```python
from build123d import *

# Parameters (mm, degrees)
SKETCH_W          = 102.2
SKETCH_H          = 83
SKETCH_W_2        = 30
SKETCH_H_2        = 5
SKETCH_W_3        = 2
SKETCH_H_3        = 25
PAD_DEPTH         = 2
SKETCH001_R       = 2.4
SKETCH001_R_2     = 1.2
PAD001_DEPTH      = 6.2
PAD002_DEPTH      = 6.9
PAD002_DEPTH_BACK = 2
PAD003_DEPTH      = 1
SKETCH004_W       = 1.45
SKETCH004_H       = 11.2
PAD004_DEPTH      = 7
SKETCH005_W       = 1.45
SKETCH005_H       = 5
PAD005_DEPTH      = 3
PAD006_DEPTH      = 5
SKETCH008_W       = 35.5
SKETCH008_H       = 1
POCKET_DEPTH      = 107.001
SKETCH009_W       = 14
SKETCH009_H       = 1
POCKET001_DEPTH   = 4.5


with BuildPart() as part:
    # Sketch → Pad (new body)
    with BuildSketch(Plane.XY):
        Rectangle(SKETCH_W, SKETCH_H)
        with Locations((34.1, 18.5)):
            Rectangle(SKETCH_W_2, SKETCH_H_2, mode=Mode.SUBTRACT)
        with Locations((6, -27)):
            Rectangle(SKETCH_W_3, SKETCH_H_3, mode=Mode.SUBTRACT)
        with Locations((-34.1, 18.5)):
            Rectangle(SKETCH_W_2, SKETCH_H_2, mode=Mode.SUBTRACT)
        with Locations((-6, -27)):
            Rectangle(SKETCH_W_3, SKETCH_H_3, mode=Mode.SUBTRACT)
    extrude(amount=PAD_DEPTH)

    # Sketch001 (on Face22 of Pad) → Pad001 (join)
    with BuildSketch(Plane.XY.offset(2)):
        with Locations((-42.5, -25)):
            Circle(SKETCH001_R)
        with Locations((-42.5, -25)):
            Circle(SKETCH001_R_2, mode=Mode.SUBTRACT)
        with Locations((42.5, 25)):
            Circle(SKETCH001_R)
        with Locations((42.5, 25)):
            Circle(SKETCH001_R_2, mode=Mode.SUBTRACT)
    extrude(amount=PAD001_DEPTH)

    # Sketch002 (on Face5 of Pad001) → Pad002 (join, two sides)
    with BuildSketch(Plane.XY.offset(2)) as pad002_sk:
        Polygon((51.1, 5), (53.5, 5), (53.5, 43.85), (-53.5, 43.85), (-53.5, 5), (-51.1, 5), (-51.1, 41.5), (51.1, 41.5), align=None)
        Polygon((51.1, -5), (53.5, -5), (53.5, -43.85), (-53.5, -43.85), (-53.5, -5), (-51.1, -5), (-51.1, -41.5), (51.1, -41.5), align=None)
    extrude(amount=PAD002_DEPTH)
    extrude(pad002_sk.sketch, amount=-PAD002_DEPTH_BACK)

    # Sketch003 (on Face33 of Pad002) → Pad003 (join)
    with BuildSketch(Plane.XY.offset(8.9)):
        Polygon((-52.1, 5), (-51.1, 5), (-51.1, 41.5), (51.1, 41.5), (51.1, 5), (52.1, 5), (52.1, 42.5), (-52.1, 42.5), align=None)
        Polygon((-52.1, -5), (-51.1, -5), (-51.1, -41.5), (51.1, -41.5), (51.1, -5), (52.1, -5), (52.1, -42.5), (-52.1, -42.5), align=None)
    extrude(amount=PAD003_DEPTH)

    # Sketch004 (on Face3 of Pad003) → Pad004 (join)
    with BuildSketch(Plane.XY.offset(2)):
        with Locations((50.375, 0)):
            Rectangle(SKETCH004_W, SKETCH004_H)
        with Locations((-50.375, 0)):
            Rectangle(SKETCH004_W, SKETCH004_H)
    extrude(amount=PAD004_DEPTH)

    # Sketch005 (on Face49 of Pad004) → Pad005 (join)
    with BuildSketch(Plane.XY.offset(9)):
        with Locations((50.375, 0)):
            Rectangle(SKETCH005_W, SKETCH005_H)
        with Locations((-50.375, 0)):
            Rectangle(SKETCH005_W, SKETCH005_H)
    extrude(amount=PAD005_DEPTH)

    # Sketch006 (on Face45 of Pad005) → Pad006 (join)
    with BuildSketch(Plane.XZ.offset(2.5)):
        Polygon((-51.10001, 12), (-53.10001, 12), (-53.10001, 13), (-51.15, 16), (-49.65, 16), (-49.65, 12), align=None)
    pad006 = extrude(amount=-PAD006_DEPTH)

    # Mirrored: Pad006 across YZ
    add(pad006.mirror(Plane.YZ))

    # Sketch008 (on Face47 of Mirrored) → Pocket (cut, through all)
    with BuildSketch(Plane.YZ.offset(53.5)):
        with Locations((0, 0.5)):
            Rectangle(SKETCH008_W, SKETCH008_H)
    extrude(amount=-POCKET_DEPTH, mode=Mode.SUBTRACT)

    # Sketch009 (on Face74 of Pocket) → Pocket001 (cut)
    with BuildSketch(Plane.XZ.offset(43.85)):
        with Locations((0, 0.5)):
            Rectangle(SKETCH009_W, SKETCH009_H)
    extrude(amount=-POCKET001_DEPTH, mode=Mode.SUBTRACT)


solid = part.part
```
Read the model definition and answer for the solid it produces. Units are mm, in the model's axes. A direction names the side the tool comes from. Coordinates: 2 decimals unless noted, no trailing zeros. Write each loop counter-clockwise with the first axis right and the second up, starting at its lowest first coordinate (ties: lowest second). Pieces come first, ordered by that corner, then holes. Notation, with made-up numbers: (-19, 5.25) - (38, 5.25) arc R11 cw to (38, 22.25) - close; hole circle Ø1 at (41.5, 35.25). An arc over 180 degrees is marked (long way). Answer as a JSON object with one key per item and string values. Group by question number.
1. A cutting plane is placed at D-D (x = -17.5). Determine the outline of the cut face in (y, z).
2. A cutting plane is placed at B-B (y = -20). Determine the outline of the cut face in (x, z).
3. Which of the six approach directions +Z, -Z, +X, -X, +Y, -Y give full straight-line access (tool end or side, diameter ignored) to faces 1 (the flat face through (1, 0, 1)), 2 (the flat face through (52, -5, 6)), 3 (the flat face through (0, -42, 1)), 4 (the flat face through (51.1, 0, 6)), 5 (the flat face through (41, 25, 8.2))?
4. Consider L1, parallel to Y at x = 42.5, z = 6.25; L2, parallel to Y at x = 19, z = 4.5; L3, parallel to Y at x = 34, z = 9.5. Determine where each line is inside the solid, lowest interval first. Write a range as [from, to].
5. The mould has two halves that part along Y. Classify faces 6 (the flat face through (51.1, -24, 6)), 7 (the flat face through (-31, -31, 0)), 8 (the flat face through (1, -43.85, 5)): +Y half, -Y half, draft (parallel to the pull), parting line (faces both ways), or undercut.
6. Each of these flat-tipped pins is pushed along its axis until it touches: P1, Ø0.8, axis at y = 16, z = 9.5, coming from the -X side; P2, Ø2, axis at x = 52.5, y = 1, coming from the -Z side; P3, Ø5.5, axis at y = -1.5, z = 7.5, coming from the -X side. Where does it stop, or does it pass through?
7. A cutting plane is placed at C-C (x = 42.5). Determine the outline of the cut face in (y, z), plus the area to 3 significant figures.
8. A cutting plane is placed at A-A (z = 7). Determine the outline of the cut face in (x, y).
Worked out:
{
 "1": {"outline": "(-43.85, 0) - (-17.75, 0) - (-17.75, 1) - (17.75, 1) - (17.75, 0) - (43.85, 0) - (43.85, 8.9) - (42.5, 8.9) - (42.5, 9.9) - (41.5, 9.9) - (41.5, 2) - (-41.5, 2) - (-41.5, 9.9) - (-42.5, 9.9) - (-42.5, 8.9) - (-43.85, 8.9) - close"},
 "2": {"outline": "(-53.5, 0) - (-7, 0) - (-7, 2) - (-51.1, 2) - (-51.1, 9.9) - (-52.1, 9.9) - (-52.1, 8.9) - (-53.5, 8.9) - close; (-5, 0) - (5, 0) - (5, 2) - (-5, 2) - close; (7, 0) - (53.5, 0) - (53.5, 8.9) - (52.1, 8.9) - (52.1, 9.9) - (51.1, 9.9) - (51.1, 2) - (7, 2) - close"},
 "3": {"face 1": "-Z, +X, -X", "face 2": "+Z, -Z, +X", "face 3": "-Z, -Y", "face 4": "-Z, +X", "face 5": "+Z"},
 "4": {"L1": "y = [-43.85, -41.5], [22.6, 23.8], [26.2, 27.4], [41.5, 43.85]", "L2": "y = [-43.85, -41.5], [41.5, 43.85]", "L3": "y = [-42.5, -41.5], [41.5, 42.5]"},
 "5": {"face 6": "undercut", "face 7": "draft", "face 8": "-Y half"},
 "6": {"P1": "stops at x = -52.1", "P2": "stops at z = 12", "P3": "stops at x = -51.1"},
 "7": {"outline": "(-43.85, 0) - (-17.75, 0) - (-17.75, 1) - (16, 1) - (16, 2) - (-41.5, 2) - (-41.5, 9.9) - (-42.5, 9.9) - (-42.5, 8.9) - (-43.85, 8.9) - close; (21, 0) - (43.85, 0) - (43.85, 8.9) - (42.5, 8.9) - (42.5, 9.9) - (41.5, 9.9) - (41.5, 2) - (27.4, 2) - (27.4, 8.2) - (26.2, 8.2) - (26.2, 2) - (23.8, 2) - (23.8, 8.2) - (22.6, 8.2) - (22.6, 2) - (21, 2) - close", "area": "181 mm²"},
 "8": {"outline": "(-53.5, -43.85) - (53.5, -43.85) - (53.5, -5) - (51.1, -5) - (51.1, 5) - (53.5, 5) - (53.5, 43.85) - (-53.5, 43.85) - (-53.5, 5) - (-51.1, 5) - (-51.1, -5) - (-53.5, -5) - close; circle Ø4.8 at (-42.5, -25); circle Ø4.8 at (42.5, 25); hole (-51.1, -41.5) - (51.1, -41.5) - (51.1, -5.6) - (49.65, -5.6) - (49.65, 5.6) - (51.1, 5.6) - (51.1, 41.5) - (-51.1, 41.5) - (-51.1, 5.6) - (-49.65, 5.6) - (-49.65, -5.6) - (-51.1, -5.6) - close; hole circle Ø2.4 at (-42.5, -25); hole circle Ø2.4 at (42.5, 25)"}
}
